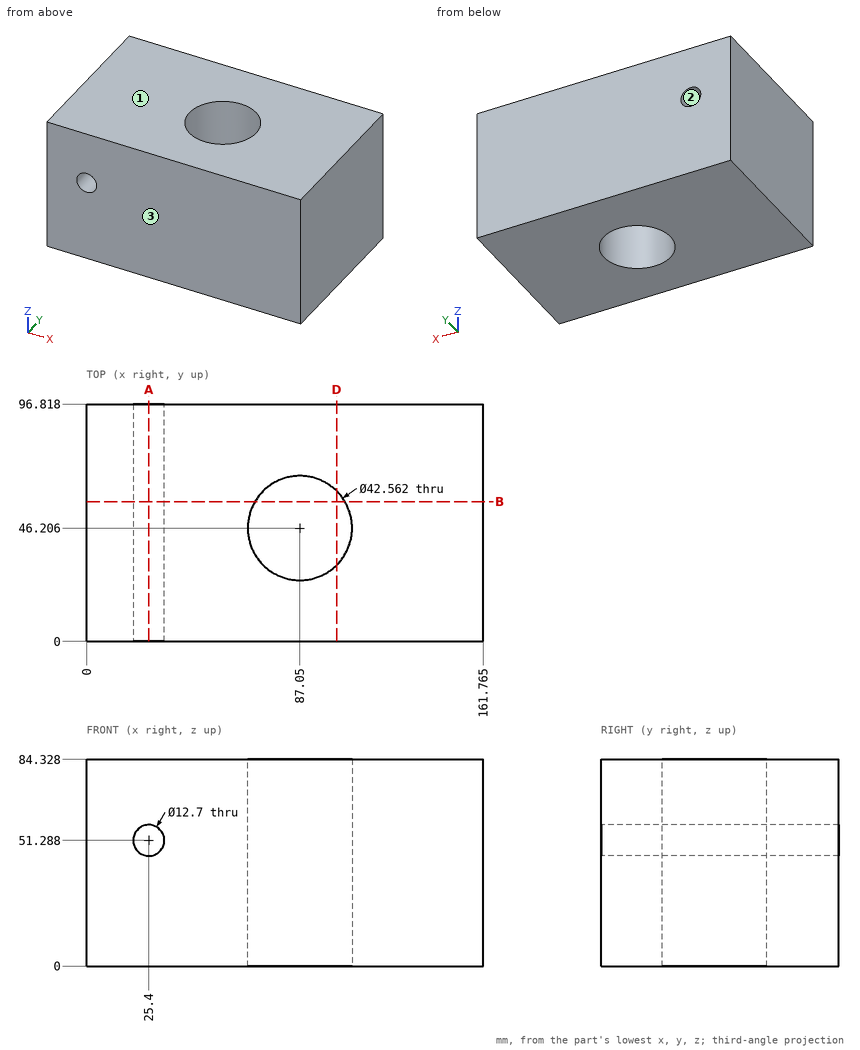
Answer from the drawing. Dimensions are ordinates in mm from the lowest x, y and z of the part. Round coordinates to 2 decimals unless told otherwise and drop trailing zeros. Write each loop counter-clockwise with the first axis right and the second up, starting at its lowest first coordinate (ties: lowest second). Pieces come first, ordered by that corner, then holes. Notation, with made-up numbers: M 57,54 L 107,54 A21 ccw 107,65 Z; hole C 9,6 d8. An arc over 180 degrees is marked long. One line per item, written item: value.
Q1. Straight lines are drawn through the part: line 1 (Z direction, x = 25.4, y = 51); line 2 (X direction, y = 32, z = 21.5) (1 decimal); line 3 (Y direction, x = 86.5, z = 16). For each, find the intervals that lie inside material, in ascending order. Write a range as [from, to].
Data:
line 1: [0, 44.94], [57.64, 84.33]
line 2: [0, 71.2], [102.9, 161.8]
line 3: [0, 24.93], [67.48, 96.82]
Q2. Find section A-A on x = 25.4. Write down the section's boundary in (y, z).
Data:
outline: M 0,0 L 96.82,0 L 96.82,44.94 L 0,44.94 Z; M 0,57.64 L 96.82,57.64 L 96.82,84.33 L 0,84.33 Z
Q3. Find section D-D on x = 102. Write down the section's boundary in (y, z).
Data:
outline: M 0,0 L 31.06,0 L 31.06,84.33 L 0,84.33 Z; M 61.35,0 L 96.82,0 L 96.82,84.33 L 61.35,84.33 Z
Q4. Flat-ended cylindrical pins translate along their axes: pin 1 Ø4 at (x, z) = (21, 33.5) entering from -Y; pin 2 Ø7.5 at (x, z) = (25.4, 51.29) entering from -Y. Find the tip coordinate at first contact, or state that the pin passes through.
Data:
pin 1: y = 0
pin 2: through
Q5. For a pull along Z with two mould halves and no side action, classify the marked faces 1, 2 and 3 as +Z half, -Z half, draft (parallel to the pull), parting line (faces both ways), or undercut.
Data:
face 1: +Z half
face 2: undercut
face 3: draft
Q6. Find section B-B on y = 57. Count the separate pieces of the cut face and the enclosed holes in it, plus the area to 3 significant figures.
Data:
separate pieces: 2
enclosed holes: 1
area: 10,400 mm2
